```python
from build123d import *

# Parameters (mm, degrees)
F1_DEPTH  = 34
F9_W      = 6
F9_H      = 24
F10_DEPTH = 10
F11_W     = 6
F11_H     = 24
F12_DEPTH = 10
F13_R     = 5


with BuildPart() as f1:
    # F0 (on Top) → F1 (new body)
    with BuildSketch(Plane.XY):
        with BuildLine():
            Line((-15, 14), (-11.313708, 14))
            ThreePointArc((-11.313708, 14), (0, -18), (11.313708, 14))
            Line((11.313708, 14), (15, 14))
            Line((15, 14), (15, 17))
            Line((15, 17), (-15, 17))
            Line((-15, 17), (-15, 14))
        make_face()
        with BuildLine():
            ThreePointArc((5.385165, 14), (0, -15), (-5.385165, 14))
            Line((-5.385165, 14), (5.385165, 14))
        make_face(mode=Mode.SUBTRACT)
    extrude(amount=F1_DEPTH)

    # F9 (on face) → F10 (cut)
    with BuildSketch(Plane(origin=(-15.588457, -9, 0), x_dir=(0.5, -0.866025, 0), z_dir=(-0.866025, -0.5, 0))):
        with Locations((-3, 17)):
            Rectangle(F9_W, F9_H)
        with Locations((3, 17)):
            Rectangle(F9_W, F9_H)
    extrude(amount=-F10_DEPTH, mode=Mode.SUBTRACT)

    # F11 (on face) → F12 (cut)
    with BuildSketch(Plane(origin=(15.588457, -9, 0), x_dir=(0.5, 0.866025, 0), z_dir=(0.866025, -0.5, 0))):
        with Locations((-3, 17)):
            Rectangle(F11_W, F11_H)
        with Locations((3, 17)):
            Rectangle(F11_W, F11_H)
    extrude(amount=-F12_DEPTH, mode=Mode.SUBTRACT)

    # F13
    f13_edges = [f1.edges().sort_by_distance(p)[0] for p in [
        (16.30141, -2.48342, 29),
        (10.30141, -12.875725, 29),
        (-16.30141, -2.48342, 29),
        (-10.30141, -12.875725, 29),
    ]]
    fillet(f13_edges, radius=F13_R)


solid = f1.part
```
Work out the finished part from the listing and answer in its coordinate system (mm). A direction names the side the tool comes from. Coordinates: 2 decimals unless noted, no trailing zeros. Loops run counter-clockwise (first coordinate to the right, second up) from the corner with the lowest first, then second, coordinate; pieces in that order, holes last.
1) Consider probe 1 along Y at (x, z) = (0, 18); probe 2 along X at (y, z) = (0, 21); probe 3 along X at (y, z) = (-9, 30). Determine where each line is inside the solid, lowest interval first.
Results:
probe 1: y = -18 to -15, 14 to 17
probe 2: x = -18 to -15, 15 to 18
probe 3: x = -15.59 to -12, 12 to 15.59
2) Flat-ended cylindrical pins translate along their axes: pin 1 (2.5 mm diameter, centred on x = -11.5, y = -6.5, fed in from +Z); pin 2 (8.5 mm diameter, centred on x = 1.5, z = 13.5, fed in from -Y); pin 3 (1.5 mm diameter, centred on y = 3.5, z = 23, fed in from +X); pin 4 (3.5 mm diameter, centred on y = 16, z = 20, fed in from -X). Find the tip coordinate at first contact, or state that the pin passes through.
Results:
pin 1: passes through
pin 2: stops at y = -18
pin 3: stops at x = 17.79
pin 4: stops at x = -15
3) Section B-B (z = 31) is taken. Give the vertices of the cut face in (x, y), plus the area to 3 significant figures.
Results:
outline: (-15, 14) - (-11.31, 14) arc R18 ccw (long way) to (11.31, 14) - (15, 14) - (15, 17) - (-15, 17) - close; hole (-5.39, 14) arc R15 ccw (long way) to (5.39, 14) - close
area: 346 mm2
4) Section C-C (y = 0) is taken. Give the vertices of the cut face in (x, z), plus the area to 3 significant figures.
Results:
outline: (-18, 0) - (-15, 0) - (-15, 34) - (-18, 34) - close; (15, 0) - (18, 0) - (18, 34) - (15, 34) - close
area: 204 mm2
5) Section A-A (x = 0) is taken. Give the vertices of the cut face in (y, z).
Results:
outline: (-18, 0) - (-15, 0) - (-15, 34) - (-18, 34) - close; (14, 0) - (17, 0) - (17, 34) - (14, 34) - close
6) For faces 4 (the flat face through (16.321, -2.495, 14.367)), 5 (the flat face through (0, 14, 17)), 6 (the cylindrical face through (11.5, -11.8, 27.6)), 7 (the flat face through (-14, -8, 29)), determine the directions among +Z, -Z, +X, -X, +Y, -Y from which every point of the face is accessible in a straight line to the end or side of a thin tool.
Results:
face 4: -Y
face 5: +Z, -Z
face 6: +X
face 7: none
7) Section D-D (z = 27.5) is taken. Give the vertices of the cut face in (x, y), plus the area to 3 significant figures.
Results:
outline: (-17.36, -4.75) - (-14.66, -3.18) arc R15 cw to (-5.39, 14) - (5.39, 14) arc R15 cw to (14.66, -3.18) - (17.36, -4.75) arc R18 ccw to (11.31, 14) - (15, 14) - (15, 17) - (-15, 17) - (-15, 14) - (-11.31, 14) arc R18 ccw to start; (-12.79, -12.66) arc R18 ccw to (12.79, -12.66) - (10.09, -11.1) arc R15 cw to (-10.09, -11.1) - close
area: 291 mm2
8) For a pull along Y with two mould halves and no side action, classify faces 1 (the flat face through (-15, 16, 17)), 2 (the flat face through (13, 14, 17)), 3 (the flat face through (0, 17, 17)) as +Y half, -Y half, draft (parallel to the pull), parting line (faces both ways), or undercut.
Results:
face 1: draft
face 2: undercut
face 3: +Y half
